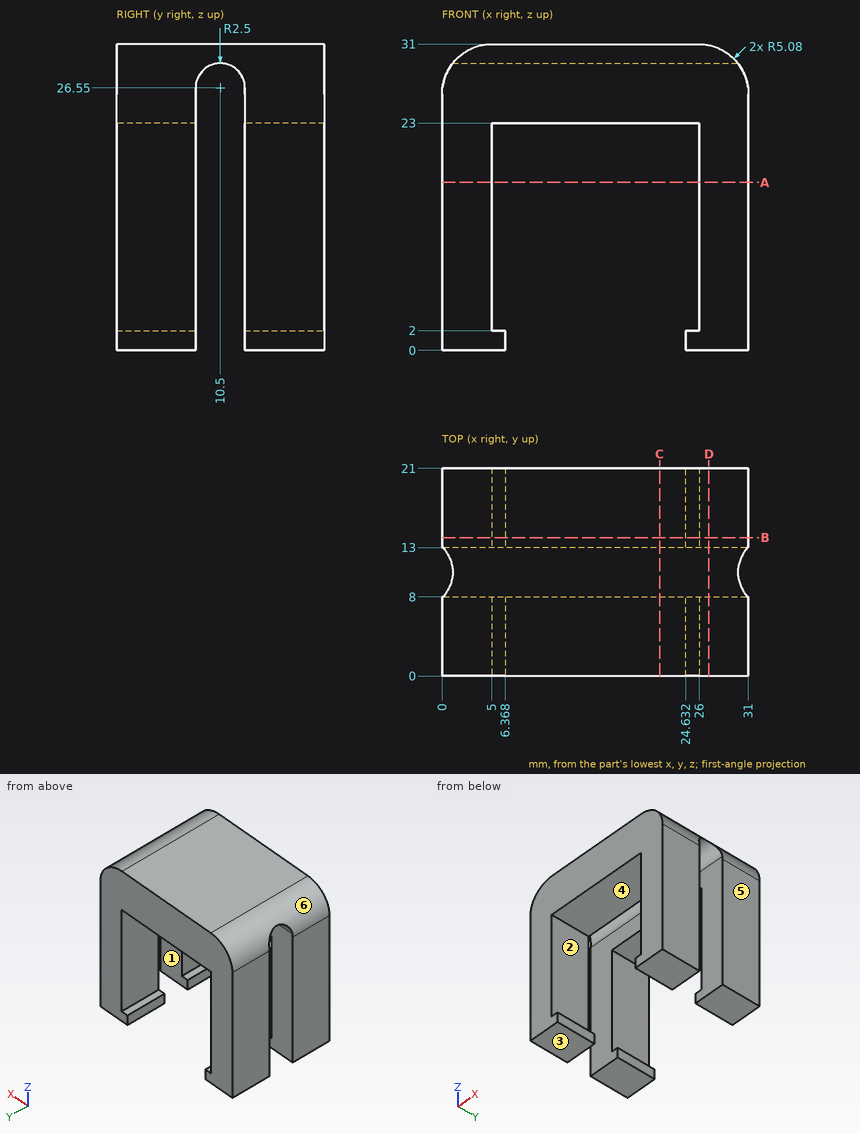
Job drawing, mm, ordinate dimensions from the low corner. One solid piece. A direction names the side the tool comes from. Round coordinates to 2 decimals unless told otherwise and drop trailing zeros. Loops run counter-clockwise (first coordinate to the right, second up) from the corner with the lowest first, then second, coordinate; pieces in that order, holes last.
Item 1: Cut at B-B, the plane y = 14. Give the cut face in (x, z), then the cut area to 3 significant figures.
Item 2: Drill centre lines: line 1 (X direction, y = 2.75, z = 12); line 2 (Y direction, x = 29, z = 26); line 3 (Z direction, x = 12.5, y = 18.5). Where is each one in solid material? Low to high.
Item 3: Drop flat-ended pins along their axis: P1, Ø4, axis at x = 16, y = 4, coming from the -Z side; P2, Ø4, axis at y = 6, z = 27, coming from the -X side. Give the stop position or say it passes through.
Item 4: Cut at A-A, the plane z = 17. Give the cut face in (x, y), then the cut area to 3 significant figures.
Item 5: Cut at D-D, the plane x = 27. Give the cut face in (y, z).
Item 6: 3-axis set-ups, long thin cutter, end or side, ignore diameter. For the marked faces 1, 2 and 3: which of +Z, -Z, +X, -X, +Y, -Y reach the whole face in a straight line?
Item 7: Mould opens along X. For the marked faces 4, 5 and 6 say: +X half, -X half, draft (parallel to the pull), parting line (faces both ways), or undercut.
Item 8: Cut at C-C, the plane x = 22. Give the cut face in (y, z), then the cut area to 3 significant figures.
A:
1. outline: (0, 0) - (6.37, 0) - (6.37, 2) - (5, 2) - (5, 23) - (26, 23) - (26, 2) - (24.63, 2) - (24.63, 0) - (31, 0) - (31, 25.92) arc R5.08 ccw to (25.92, 31) - (5.08, 31) arc R5.08 ccw to (0, 25.92) - close
1. area: 472 mm2
2. line 1: x = 0 to 5, 26 to 31
2. line 2: y = 0 to 8, 13 to 21
2. line 3: z = 23 to 31
3. P1: stops at z = 23
3. P2: stops at x = 0
4. outline: (0, 0) - (5, 0) - (5, 8) - (0, 8) - close; (0, 13) - (5, 13) - (5, 21) - (0, 21) - close; (26, 0) - (31, 0) - (31, 8) - (26, 8) - close; (26, 13) - (31, 13) - (31, 21) - (26, 21) - close
4. area: 160 mm2
5. outline: (0, 0) - (8, 0) - (8, 26.55) arc R2.5 cw to (13, 26.55) - (13, 0) - (21, 0) - (21, 30.88) - (0, 30.88) - close
6. face 1: -Z, +X, -X
6. face 2: +Y, -Y
6. face 3: -Z, +X, -X, +Y, -Y
7. face 4: undercut
7. face 5: +X half
7. face 6: -X half
8. outline: (0, 23) - (8, 23) - (8, 26.55) arc R2.5 cw to (13, 26.55) - (13, 23) - (21, 23) - (21, 31) - (0, 31) - close
8. area: 140 mm2
